Geometry check sheet. Reference: the model listing, model coordinates, mm. A direction names the side the tool comes from. Give positions to 0.01 mm unless a question says otherwise; leave off trailing zeros. Order: outer loops, then holes, each group sorted by start corner. A loop starts at its lowest first (then second) coordinate and runs counter-clockwise, first axis right, second up. Notation, with made-up numbers: M 65.25,-27 L 75.25,-27 A31 ccw 75.25,8 Z; hole C 47.5,75 d4. An arc over 180 degrees is marked long. Put each result on its own line as item: value. Start each with the question number.
Q1. Go/stop test with flat-tipped pins: pin 1 (3 mm diameter, centred on y = 9, z = -15, fed in from +X); pin 2 (1.5 mm diameter, centred on x = 21, y = 10, fed in from -Z); pin 3 (1 mm diameter, centred on y = 10.5, z = -6, fed in from +X). Record where each tip stops, or that it passes through.
Q2. Access from +Z, -Z, +X, -X, +Y, -Y to the whole of each face (thin tool, end or side, straight path). Record for faces 1 (the flat face through (21, 9, -4)), 2 (the cylindrical face through (3.04, 14.09, -10.4)).
Q3. Material ranges on L1, parallel to Y at x = 25, z = -1.3; L2, parallel to Z at x = 3.05, y = 4; L3, parallel to Y at x = 1.75, z = -12.5, recorded low to high.
Q4. Mould release check, pull along X, two halves, no side actions. Record for faces 3 (the cylindrical face through (7, 9.13, -5.05)), 4 (the cylindrical face through (17.926, 7.372, -1.972)), 5 (the flat face through (8, 18, -3)): +X half, -X half, draft (parallel to the pull), parting line (faces both ways), or undercut.
Q5. Section check C-C on x = 14. Record the cut outline in (y, z), then the cut area to 3 significant figures.
Q6. Section check D-D on x = 2.75. Record the cut outline in (y, z), then the cut area to 3 significant figures.
Q7. Section check A-A on y = 9. Record the cut outline in (x, z).
Q8. Section check B-B on z = -12.5. Record the cut outline in (x, y), then the cut area to 3 significant figures.
```python
from build123d import *

# Parameters (mm, degrees)
BOSS_EXTRUDE1_DEPTH = 18
SKETCH4_R           = 1.6
CUT_EXTRUDE2_DEPTH  = 38.841775857
FILLET1_R           = 3.5
SKETCH7_R           = 2.1
CUT_EXTRUDE5_DEPTH  = 6
SKETCH8_R           = 4.25
CUT_EXTRUDE6_DEPTH  = 38.841775857


with BuildPart() as part:
    # Sketch1 → Boss-Extrude1 (new body)
    with BuildSketch(Plane(origin=(0, 0, 0), x_dir=(1, 0, 0), z_dir=(0, 1, 0))):
        Polygon((0, 18), (0, 0), (28, 0), (28, 4), (6, 4), (6, 18), align=None)
    extrude(amount=BOSS_EXTRUDE1_DEPTH)

    # Sketch4 → Cut-Extrude2 (cut, through all)
    with BuildSketch(Plane.XY):
        with Locations((25, 9)):
            Circle(SKETCH4_R)
        with Locations((3, 9)):
            Circle(SKETCH4_R)
    extrude(amount=-CUT_EXTRUDE2_DEPTH, mode=Mode.SUBTRACT)

    # Fillet1
    fillet1_edges = [part.edges().sort_by_distance(p)[0] for p in [
        (6, 9, -4),
    ]]
    fillet(fillet1_edges, radius=FILLET1_R)

    # Sketch7 → Cut-Extrude5 (cut)
    with BuildSketch(Plane(origin=(6, 0, 0), x_dir=(0, 0, -1), z_dir=(1, 0, 0))):
        with Locations((12.5, 14)):
            Circle(SKETCH7_R)
        with Locations(Location((12.5, 4, 0), (0, 0, 180))):
            Circle(SKETCH7_R)
    extrude(amount=-CUT_EXTRUDE5_DEPTH, mode=Mode.SUBTRACT)

    # Sketch8 → Cut-Extrude6 (cut, through all)
    with BuildSketch(Plane.XY):
        with Locations((14, 9)):
            Circle(SKETCH8_R)
    extrude(amount=-CUT_EXTRUDE6_DEPTH, mode=Mode.SUBTRACT)


solid = part.part
```
Results found:
1. pin 1: stops at x = 6
1. pin 2: stops at z = -4
1. pin 3: stops at x = 6.63
2. face 1: -Z, +X, +Y, -Y
2. face 2: +X, -X
3. L1: y = 0 to 7.4, 10.6 to 18
3. L2: z = -18 to -14.6, -10.4 to 0
3. L3: y = 0 to 1.9, 6.1 to 8, 10 to 11.9, 16.1 to 18
4. face 3: +X half
4. face 4: undercut
4. face 5: draft
5. outline: M 0,-4 L 4.75,-4 L 4.75,0 L 0,0 Z; M 13.25,-4 L 18,-4 L 18,0 L 13.25,0 Z
5. area: 38.0 mm^2
6. outline: M 0,-18 L 7.42,-18 L 7.42,0 L 0,0 Z; M 10.58,-18 L 18,-18 L 18,0 L 10.58,0 Z; hole C 4,-12.5 d4.2; hole C 14,-12.5 d4.2
6. area: 239 mm^2
7. outline: M 0,-18 L 1.4,-18 L 1.4,0 L 0,0 Z; M 4.6,-18 L 6,-18 L 6,-7.5 A3.5 cw 9.5,-4 L 9.75,-4 L 9.75,0 L 4.6,0 Z; M 18.25,-4 L 23.4,-4 L 23.4,0 L 18.25,0 Z; M 26.6,-4 L 28,-4 L 28,0 L 26.6,0 Z
8. outline: M 0,0 L 6,0 L 6,1.9 L 0,1.9 Z; M 0,6.1 L 6,6.1 L 6,11.9 L 0,11.9 Z; M 0,16.1 L 6,16.1 L 6,18 L 0,18 Z; hole C 3,9 d3.2
8. area: 49.6 mm^2
